Read the model definition and answer for the solid it produces. Units are mm, in the model's axes. A direction names the side the tool comes from. Give positions to 0.01 mm unless a question says otherwise; leave off trailing zeros. Write each loop counter-clockwise with the first axis right and the second up, starting at its lowest first coordinate (ties: lowest second). Pieces come first, ordered by that corner, then holes. Notation, with made-up numbers: (-7, 84.25) -> (11, 84.25) arc R25 cw to (11, 120.25) -> close; hole circle Ø10 at (-31.5, 46). An arc over 180 degrees is marked (long way). Use a Markdown table: item, result.
from build123d import *

# Parameters (mm, degrees)
PAD_DEPTH         = 10
SKETCH001_W       = 20
SKETCH001_H       = 10
PAD001_DEPTH      = 10
SKETCH002_R       = 5
POCKET_DEPTH      = 18.501
POCKET_DEPTH_BACK = -18.501


with BuildPart() as part:
    # Sketch → Pad (new body)
    with BuildSketch(Plane.XZ):
        with BuildLine():
            Line((0, 5), (50, 5))
            ThreePointArc((85.406059, 5.716814), (67.437048, 18.49621), (50, 5))
            Line((85.406059, 5.716814), (82.552889, 4.789763))
            ThreePointArc((82.552889, 4.789763), (52.311513, 0), (82.552889, -4.789763))
            Line((85.406059, -5.716814), (82.552889, -4.789763))
            ThreePointArc((50, -5), (67.437048, -18.49621), (85.406059, -5.716814))
            Line((0, -5), (50, -5))
            Line((0, 5), (0, -5))
        make_face()
    pad = extrude(amount=PAD_DEPTH)

    # Sketch001 → Pad001 (join)
    with BuildSketch(Plane.XZ):
        with Locations((10, 0)):
            Rectangle(SKETCH001_W, SKETCH001_H)
    pad001 = extrude(amount=-PAD001_DEPTH)

    # Mirrored: Pad, Pad001 across Sketch V_Axis
    add(pad.mirror(Plane(origin=(0, 0, 0), x_dir=(0, -1, 0), z_dir=(1, 0, 0))))
    add(pad001.mirror(Plane(origin=(0, 0, 0), x_dir=(0, -1, 0), z_dir=(1, 0, 0))))

    # Sketch002 → Pocket (cut, two sides)
    with BuildSketch(Plane.XY) as pocket_sk:
        Circle(SKETCH002_R)
    extrude(amount=-POCKET_DEPTH, mode=Mode.SUBTRACT)
    extrude(pocket_sk.sketch, amount=-POCKET_DEPTH_BACK, mode=Mode.SUBTRACT)


solid = part.part
Item 1: For a pull along Y with two mould halves and no side action, classify faces 1 (the face through (0, 10, 0)), 2 (the face through (-1.08, -4.88, 0.07)), 3 (the face through (1, -7, -5)), 4 (the face through (0, -10, -1)) as +Y half, -Y half, draft (parallel to the pull), parting line (faces both ways), or undercut.
Return value:
| item | result |
|---|---|
| face 1 | +Y half |
| face 2 | undercut |
| face 3 | draft |
| face 4 | -Y half |
Item 2: A tool of negligible diameter and unlimited length cuts with its end or side. For faces 5 (the face through (84, -4.93, 5.26)), 6 (the face through (-84, -4.93, 5.26)), 7 (the face through (-20, 5, 0)), 8 (the face through (20, 5, 0)), 9 (the face through (1, -7, 5)), from which of +Z, -Z, +X, -X, +Y, -Y can it reach the whole face along a straight path? Write none if from no direction.
Return value:
| item | result |
|---|---|
| face 5 | +X, +Y, -Y |
| face 6 | -X, +Y, -Y |
| face 7 | +Z, -Z, -X, +Y |
| face 8 | +Z, -Z, +X, +Y |
| face 9 | +Z, +Y, -Y |
Item 3: A cutting plane is placed at D-D (x = 39). Give the vertices of the cut face in (y, z).
Return value:
| item | result |
|---|---|
| outline | (-10, -5) -> (0, -5) -> (0, 5) -> (-10, 5) -> close |
Item 4: Each of these flat-tipped pins is pushed along its axis until it touches: P1, Ø4, axis at x = 66, y = -7, coming from the -Z side; P2, Ø8, axis at y = 6.5, z = -2, coming from the -X side; P3, Ø2, axis at x = -5, y = 7, coming from the +Z side; P4, Ø18.5, axis at x = -37, z = -8, coming from the +Y side. Where does it stop, or does it pass through?
Return value:
| item | result |
|---|---|
| P1 | z = -18.5 |
| P2 | x = -20 |
| P3 | z = 5 |
| P4 | y = 0 |
Item 5: A cutting plane is placed at B-B (z = -9.5). Give the vertices of the cut face in (x, y).
Return value:
| item | result |
|---|---|
| outline | (-83.69, -10) -> (-80.06, -10) -> (-80.06, 0) -> (-83.69, 0) -> close; (-55.56, -10) -> (-51.94, -10) -> (-51.94, 0) -> (-55.56, 0) -> close; (51.94, -10) -> (55.56, -10) -> (55.56, 0) -> (51.94, 0) -> close; (80.06, -10) -> (83.69, -10) -> (83.69, 0) -> (80.06, 0) -> close |
Item 6: Straight lines are drawn through the part: line 1 along X through (y, z) = (-1.5, 1); line 2 along X through (y, z) = (0.5, -3.5); line 3 along X through (y, z) = (-6.5, -13.5). For each, find the intervals that lie inside material, in ascending order. Write a range as [from, to].
Return value:
| item | result |
|---|---|
| line 1 | [-52.34, -4.77], [4.77, 52.34] |
| line 2 | [-20, -4.97], [4.97, 20] |
| line 3 | [-80.46, -75.43], [-60.2, -55.16], [55.16, 60.2], [75.43, 80.46] |
Item 7: A cutting plane is placed at C-C (z = 0). Give the vertices of the cut face in (x, y).
Return value:
| item | result |
|---|---|
| outline | (-52.31, -10) -> (52.31, -10) -> (52.31, 0) -> (20, 0) -> (20, 10) -> (-20, 10) -> (-20, 0) -> (-52.31, 0) -> close; hole circle Ø10 at (0, 0) |
Item 8: A cutting plane is placed at A-A (x = -67.5). Give the vertices of the cut face in (y, z).
Return value:
| item | result |
|---|---|
| outline | (-10, -18.5) -> (0, -18.5) -> (0, -15.5) -> (-10, -15.5) -> close; (-10, 15.5) -> (0, 15.5) -> (0, 18.5) -> (-10, 18.5) -> close |
